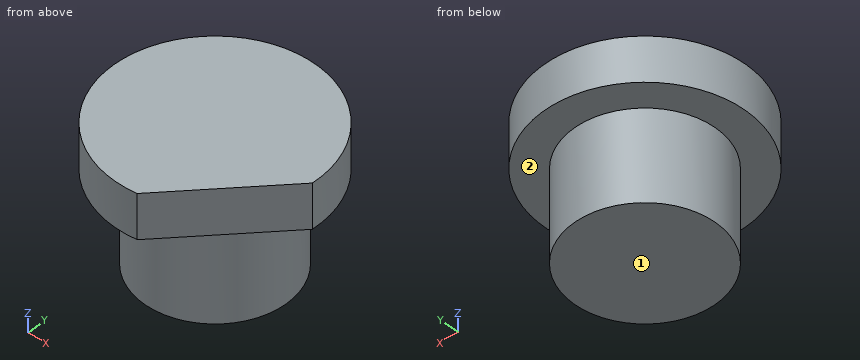
```python
from build123d import *

# Parameters (mm, degrees)
SKETCH_2_R        = 3.501329815
EXTRUDE_1_DEPTH   = 4.491890815
EXTRUDE_2_DEPTH   = 2.193354394
MOVE_BODY_1_ANGLE = 90


with BuildPart() as part:
    # Эскиз2 → Бобышка-Вытянуть1 (new body)
    with BuildSketch(Plane(origin=(0, 0, 0), x_dir=(1, 0, 0), z_dir=(0, 1, 0))):
        Circle(SKETCH_2_R)
    extrude(amount=EXTRUDE_1_DEPTH)

    # Эскиз3 → Бобышка-Вытянуть2 (add)
    with BuildSketch(Plane(origin=(0, 0, 0), x_dir=(-1, 0, 0), z_dir=(0, -1, 0))):
        with BuildLine():
            Line((-0.662486279, 4.945665231), (-4.986919029, 0.170678767))
            ThreePointArc((-4.986919029, 0.170678767), (3.698522545, -3.349540809), (-0.662486279, 4.945665231))
        make_face()
    extrude(amount=EXTRUDE_2_DEPTH)


with BuildPart() as part_1:
    # Move Body 1: moved
    add(part.part.rotate(Axis((0, 1.149268211, 0), (-1, 0, 0)), MOVE_BODY_1_ANGLE))


with BuildPart() as part_2:
    # Move Body 2: moved
    add(part_1.part.moved(Location((0, 0, -3.34))))


solid = part_2.part
```
Geometry check sheet. Reference: the model listing, model coordinates, mm. Face numbers are marked on the shaded views. A direction names the side the tool comes from. Round coordinates to 2 decimals unless told otherwise and drop trailing zeros. Loops run counter-clockwise (first coordinate to the right, second up) from the corner with the lowest first, then second, coordinate; pieces in that order, holes last. Notation, with made-up numbers: (28, -8) - (60, -8) arc R12 ccw to (60, 15) - close; hole circle Ø8 at (76.5, 31). An arc over 180 degrees is marked (long way). Use a Markdown table: item, result.
Q1. Material ranges on line 1 (Z direction, x = 1, y = 5); line 2 (Y direction, x = -0.75, z = -1.25); line 3 (Y direction, x = -2, z = -1), recorded low to high.
Solutions:
| item | result |
|---|---|
| line 1 | z = -2.19 to 0 |
| line 2 | y = -3.78 to 6.08 |
| line 3 | y = -3.42 to 5.72 |
Q2. Cross-section at B-B on y = 0.75. Record the cut outline in (x, z), plus the area to 3 significant figures.
Solutions:
| item | result |
|---|---|
| outline | (-4.97, -2.19) - (-3.48, -2.19) - (-3.48, -6.68) - (3.48, -6.68) - (3.48, -2.19) - (4.78, -2.19) - (4.78, 0) - (-4.97, 0) - close |
| area | 52.6 mm2 |
Q3. Cross-section at C-C on z = -0.25. Record the cut outline in (x, y).
Solutions:
| item | result |
|---|---|
| outline | (0.66, -3.8) - (4.99, 0.98) arc R4.99 ccw (long way) to start |
Q4. Cross-section at A-A on x = -2.5. Record the cut outline in (y, z).
Solutions:
| item | result |
|---|---|
| outline | (-3.17, -2.19) - (-1.3, -2.19) - (-1.3, -6.68) - (3.6, -6.68) - (3.6, -2.19) - (5.47, -2.19) - (5.47, 0) - (-3.17, 0) - close |
Q5. Access from +Z, -Z, +X, -X, +Y, -Y to the whole of each face (thin tool, end or side, straight path). Record for the marked faces 1 and 2.
Solutions:
| item | result |
|---|---|
| face 1 | -Z, +X, -X, +Y, -Y |
| face 2 | -Z |
Q6. Cross-section at D-D on x = -4.25. Record the cut outline in (y, z), plus the area to 3 significant figures.
Solutions:
| item | result |
|---|---|
| outline | (-1.47, -2.19) - (3.76, -2.19) - (3.76, 0) - (-1.47, 0) - close |
| area | 11.5 mm2 |
Q7. Go/stop test with flat-tipped pins: P1, Ø1.5, axis at y = 4, z = -3.5, coming from the -X side; P2, Ø1, axis at y = -0.5, z = -4, coming from the -X side; P3, Ø1, axis at y = -2.5, z = -1.5, coming from the +X side. Record where each tip stops, or that it passes through.
Solutions:
| item | result |
|---|---|
| P1 | stops at x = -2.8 |
| P2 | stops at x = -3.31 |
| P3 | stops at x = 2.29 |
